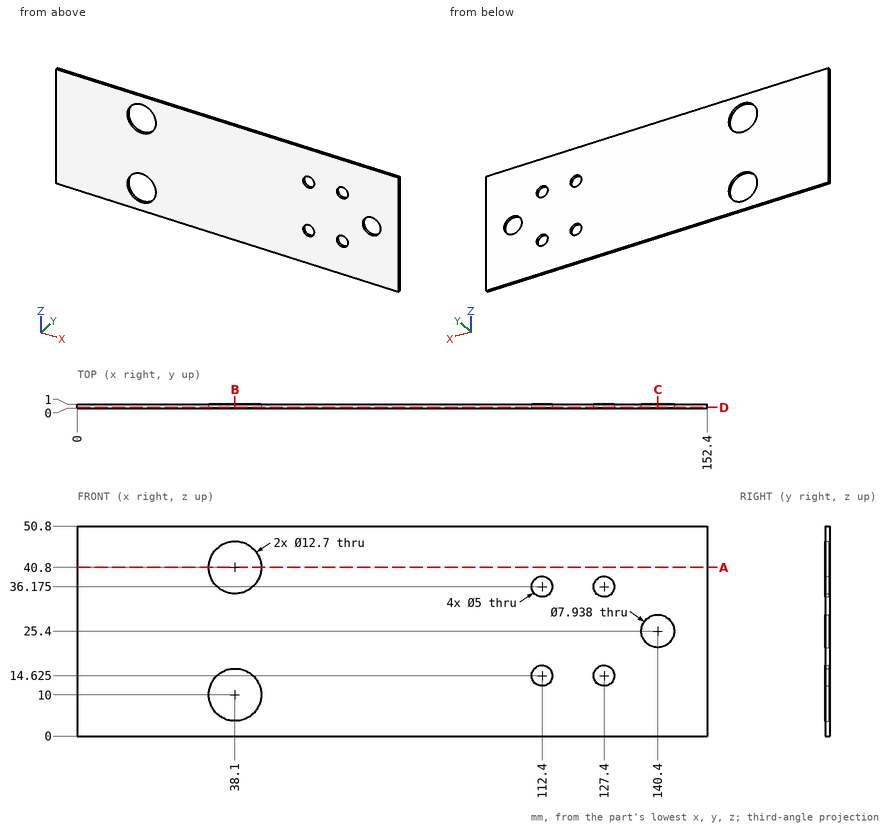
Answer from the drawing. Dimensions are ordinates in mm from the lowest x, y and z of the part. Give positions to 0.01 mm unless a question says otherwise; leave off trailing zeros. Write each loop counter-clockwise with the first axis right and the second up, starting at its lowest first coordinate (ties: lowest second). Pieces come first, ordered by that corner, then holes. Notation, with made-up numbers: (52, 58) - (111, 58) arc R18 cw to (111, 93) - close; hole circle Ø10 at (-27.75, 37). An arc over 180 degrees is marked (long way). Answer in a Markdown table with one row per item. Add a question column.
Item 1: Section D-D, the plane y = 0.2 is taken. Count the separate pieces of the cut face and the enclosed holes in it, and give its area (3 significant figures).
Item 2: Find the intervals of material crossed by L1, parallel to Z at x = 112.4, y = 0.5 (1 decimal); L2, parallel to Z at x = 38.1, y = 0.3; L3, parallel to X at y = 0.6, z = 40.5, in increasing order.
Item 3: Section B-B, the plane x = 38.1 is taken. Write down the section's boundary in (y, z).
Item 4: Section C-C, the plane x = 140.4 is taken. Write down the section's boundary in (y, z).
Item 5: Section A-A, the plane z = 40.8 is taken. Write down the section's boundary in (x, y).
Recorded:
| question | item | result |
|---|---|---|
| 1 | separate pieces | 1 |
| 1 | enclosed holes | 7 |
| 1 | area | 7,360 mm2 |
| 2 | L1 | z = 0 to 12.1, 17.1 to 33.7, 38.7 to 50.8 |
| 2 | L2 | z = 0 to 3.65, 16.35 to 34.45, 47.15 to 50.8 |
| 2 | L3 | x = 0 to 31.76, 44.44 to 152.4 |
| 3 | outline | (0, 0) - (1, 0) - (1, 3.65) - (0, 3.65) - close; (0, 16.35) - (1, 16.35) - (1, 34.45) - (0, 34.45) - close; (0, 47.15) - (1, 47.15) - (1, 50.8) - (0, 50.8) - close |
| 4 | outline | (0, 0) - (1, 0) - (1, 21.43) - (0, 21.43) - close; (0, 29.37) - (1, 29.37) - (1, 50.8) - (0, 50.8) - close |
| 5 | outline | (0, 0) - (31.75, 0) - (31.75, 1) - (0, 1) - close; (44.45, 0) - (152.4, 0) - (152.4, 1) - (44.45, 1) - close |
